Geometry: final body of the model. Coordinates: model frame, mm. Face numbers are marked on the shaded views. A direction names the side the tool comes from. Give positions to 0.01 mm unless a question says otherwise; leave off trailing zeros. Loops run counter-clockwise (first coordinate to the right, second up) from the corner with the lowest first, then second, coordinate; pieces in that order, holes last.
```python
from build123d import *

# Parameters (mm, degrees)
BODYSKETCH1_W                = 12.85
BODYSKETCH1_H                = 6.55
BODYSKETCH1_R                = 1
BODYBOSS_EXTRUDE1_DEPTH      = 2.8
SKETCH2_W                    = 1.8
SKETCH2_H                    = 13.35
LEVERBOSS_EXTRUDE2_DEPTH     = 2.5
LEVERCUT_EXTRUDE1_DEPTH      = 17.703742096
BUTTONBOSS_EXTRUDE3_REACH    = 17.574
SKETCH4_W                    = 1.8
SKETCH4_H                    = 1
SKETCH5_W                    = 0.1
SKETCH5_H                    = 1
TEREMINALBOSS_EXTRUDE4_DEPTH = 3.5


with BuildPart() as part:
    # BodySketch1 → BodyBoss-Extrude1 (new body)
    with BuildSketch(Plane(origin=(0, 0, 0), x_dir=(0, 0, -1), z_dir=(1, 0, 0))):
        with Locations((6.425, 3.275)):
            Rectangle(BODYSKETCH1_W, BODYSKETCH1_H)
        with Locations((3.25, 1.5)):
            Circle(BODYSKETCH1_R, mode=Mode.SUBTRACT)
        with Locations((9.6, 1.5)):
            Circle(BODYSKETCH1_R, mode=Mode.SUBTRACT)
    extrude(amount=BODYBOSS_EXTRUDE1_DEPTH)

    # Sketch2 → LeverBoss-Extrude2 (add)
    with BuildSketch(Plane(origin=(0, 6.55, 0), x_dir=(1, 0, 0), z_dir=(0, 1, 0))):
        with Locations((1.4, 7.175)):
            Rectangle(SKETCH2_W, SKETCH2_H)
    extrude(amount=LEVERBOSS_EXTRUDE2_DEPTH)

    # Sketch3 → LeverCut-Extrude1 (cut, through all)
    with BuildSketch(Plane(origin=(2.3, 0, 0), x_dir=(0, 0, -1), z_dir=(1, 0, 0))):
        Polygon((0.5, 6.55), (13.85, 9.05), (0.5, 9.05), align=None)
        Polygon((13.85, 8.95), (13.85, 6.55), (1.034, 6.55), align=None)
    extrude(amount=-LEVERCUT_EXTRUDE1_DEPTH, mode=Mode.SUBTRACT)

    # ButtonBoss-Extrude3: up to this plane
    buttonboss_extrude3_end = Plane(origin=(0, 6.55, -1.034), z_dir=(0, 0.982913837182172, 0.1840662616446014))
    # Sketch4 → ButtonBoss-Extrude3 (add, up to the surface)
    with BuildSketch(Plane(origin=(0, 6.55, 0), x_dir=(1, 0, 0), z_dir=(0, 1, 0)), mode=Mode.PRIVATE) as buttonboss_extrude3_sk1:
        with Locations((1.4, 4.448948019)):
            Rectangle(SKETCH4_W, SKETCH4_H)
    buttonboss_extrude3_tool1 = split(extrude(buttonboss_extrude3_sk1.sketch, amount=BUTTONBOSS_EXTRUDE3_REACH, mode=Mode.PRIVATE), bisect_by=buttonboss_extrude3_end, keep=Keep.BOTH, mode=Mode.PRIVATE)
    add(buttonboss_extrude3_tool1.solids().sort_by_distance((1.4, 6.55, -4.448948))[0])

    # Sketch5 → TereminalBoss-Extrude4 (add)
    with BuildSketch(Plane.XZ):
        with Locations((1.4, -0.7)):
            Rectangle(SKETCH5_W, SKETCH5_H)
        with Locations((1.4, -6.025)):
            Rectangle(SKETCH5_W, SKETCH5_H)
        with Locations((1.4, -12.15)):
            Rectangle(SKETCH5_W, SKETCH5_H)
    extrude(amount=TEREMINALBOSS_EXTRUDE4_DEPTH)


solid = part.part
```
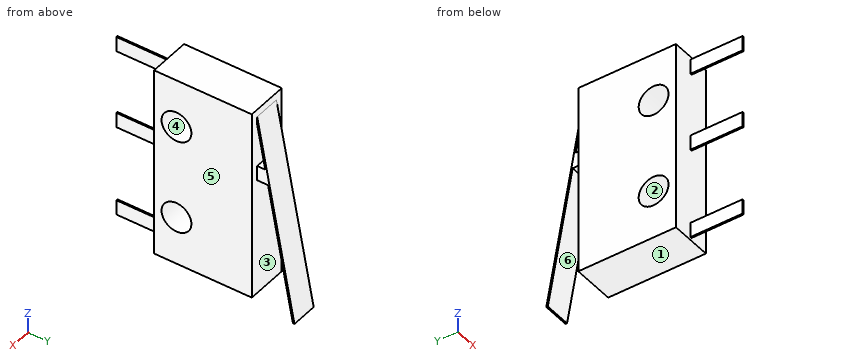
Q1. Reachability of the marked faces 1 and 2 from +Z, -Z, +X, -X, +Y, -Y: full face, straight path, thin tool, end or side. Return the list, or none.
Q2. Pin query (flat end, axial travel): pin 1 Ø0.8 at (y, z) = (-2, -0.5) entering from +X; pin 2 Ø1.5 at (x, y) = (2, 2) entering from -Z; pin 3 Ø1 at (y, z) = (-1.5, -8.5) entering from -X. Return the tip coordinate at first contact, or that it passes through.
Q3. Section query A-A, the plane y = 1.5. Return loops of the section in (x, z), and give its area (3 significant figures).
Q4. Section query C-C, the plane z = -2.75. Return loops of the section in (x, y), and give its area (3 significant figures).
Q5. Section query D-D, the plane y = 5.25. Return loops of the section in (x, z).
Q6. Section query B-B, the plane x = 1.75. Return loops of the section in (y, z).
Q7. Material intervals for probe 1 along Z at (x, y) = (0.65, 3.25), sorted ascending.
Q8. Mould query, pull axis Z, two halves, no side actions, for the marked faces 3, 4, 5 and 6. Classes: +Z half, -Z half, draft (parallel to the pull), parting line (faces both ways), or undercut.
Resolved:
1. face 1: -Z, +X, -X, -Y
1. face 2: +X, -X
2. pin 1: stops at x = 1.45
2. pin 2: stops at z = -12.85
2. pin 3: passes through
3. outline: (0, -12.85) - (2.8, -12.85) - (2.8, -10.6) - (0, -10.6) - close; (0, -8.6) - (2.8, -8.6) - (2.8, -4.25) - (0, -4.25) - close; (0, -2.25) - (2.8, -2.25) - (2.8, 0) - (0, 0) - close
3. area: 24.8 mm2
4. outline: (0, 0) - (2.8, 0) - (2.8, 0.63) - (0, 0.63) - close; (0, 2.37) - (2.8, 2.37) - (2.8, 6.55) - (0, 6.55) - close; (0.5, 6.87) - (2.3, 6.87) - (2.3, 6.97) - (0.5, 6.97) - close
4. area: 13.7 mm2
5. outline: (0, -12.85) - (2.8, -12.85) - (2.8, 0) - (0, 0) - close
6. outline: (0, -12.85) - (6.55, -12.85) - (6.55, -4.95) - (7.28, -4.95) - (8.95, -13.85) - (9.05, -13.85) - (6.55, -0.5) - (6.55, 0) - (0, 0) - close; hole circle Ø2 at (1.5, -9.6); hole circle Ø2 at (1.5, -3.25); hole (6.55, -3.95) - (7.1, -3.95) - (6.55, -1.03) - close
7. probe 1: z = -12.85 to 0
8. face 3: undercut
8. face 4: undercut
8. face 5: draft
8. face 6: -Z half
